from build123d import *

# Parameters (mm, degrees)
SKETCH1_R           = 1.25
BOSS_EXTRUDE1_DEPTH = 3


with BuildPart() as part:
    # Sketch1 → Boss-Extrude1 (new body)
    with BuildSketch(Plane.XY):
        with BuildLine():
            Line((-3.5, 0), (-3.5, -5))
            Line((-3.5, -5), (-2, -5))
            Line((-2, -5), (-2, -8))
            Line((-2, -8), (2, -8))
            Line((2, -8), (2, -5))
            Line((2, -5), (3.5, -5))
            Line((3.5, -5), (3.5, 0))
            ThreePointArc((3.5, 0), (0, 3.5), (-3.5, 0))
        make_face()
        Circle(SKETCH1_R, mode=Mode.SUBTRACT)
    extrude(amount=BOSS_EXTRUDE1_DEPTH)


solid = part.part
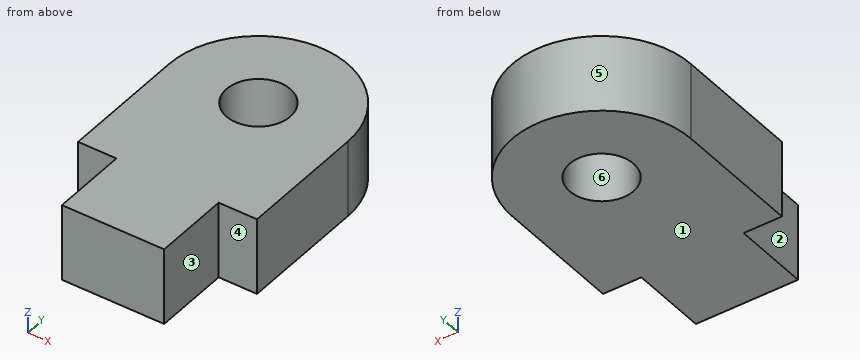
Source: CAD feature listing. Evaluate the final solid. Frame: model axes, mm. Face numbers are marked on the shaded views. A direction names the side the tool comes from. Round coordinates to 2 decimals unless told otherwise and drop trailing zeros. Order: outer loops, then holes, each group sorted by start corner. A loop starts at its lowest first (then second) coordinate and runs counter-clockwise, first axis right, second up. Notation, with made-up numbers: (82.5, 83.5) - (98.5, 83.5) arc R25 cw to (98.5, 116.5) - close; hole circle Ø7 at (-18.5, -17). An arc over 180 degrees is marked (long way). Use a Markdown table: item, result. Add a question column.
1. Mould query, pull axis X, two halves, no side actions, for the marked faces 4, 5 and 6. Classes: +X half, -X half, draft (parallel to the pull), parting line (faces both ways), or undercut.
2. Section query B-B (y = 0.25). Return the cut outline in (x, z), then the cut area to 3 significant figures.
3. Section query D-D (y = -7.25). Return the cut outline in (x, z), then the cut area to 3 significant figures.
4. Section query C-C (x = 0). Return the cut outline in (y, z), then the cut area to 3 significant figures.
5. Line query: probe 1 along Y at (x, z) = (0, 2); probe 2 along X at (y, z) = (-6, 2.05); probe 3 along Y at (x, z) = (1, 1.15). Output: solid intervals per line, ascending.
6. Section query A-A (z = 1.3). Return the cut outline in (x, y).
7. First-contact query: pin 1 (1.5 mm diameter, centred on x = -1, z = 1.5, fed in from +Y); pin 2 (1.6 mm diameter, centred on x = 2.5, z = 1, fed in from -Y); pin 3 (1.2 mm diameter, centred on x = -3, z = 1, fed in from -Y); pin 4 (1.5 mm diameter, centred on y = -6, z = 1, fed in from -X). Flat tips, straight axial feed; report the tip coordinate or a pass-through.
8. Set-up query: the marked faces 1, 2 and 3. Return all of +Z, -Z, +X, -X, +Y, -Y with unobstructed straight access to the full face (end or side cutting, diameter ignored); none if empty.
Derived:
| question | item | result |
|---|---|---|
| 1 | face 4 | draft |
| 1 | face 5 | parting line |
| 1 | face 6 | undercut |
| 2 | outline | (-3.49, 0) - (-1.22, 0) - (-1.22, 3) - (-3.49, 3) - close; (1.22, 0) - (3.49, 0) - (3.49, 3) - (1.22, 3) - close |
| 2 | area | 13.6 mm2 |
| 3 | outline | (-2, 0) - (2, 0) - (2, 3) - (-2, 3) - close |
| 3 | area | 12.0 mm2 |
| 4 | outline | (-8, 0) - (-1.25, 0) - (-1.25, 3) - (-8, 3) - close; (1.25, 0) - (3.5, 0) - (3.5, 3) - (1.25, 3) - close |
| 4 | area | 27.0 mm2 |
| 5 | probe 1 | -8 to -1.25, 1.25 to 3.5 |
| 5 | probe 2 | -2 to 2 |
| 5 | probe 3 | -8 to -0.75, 0.75 to 3.35 |
| 6 | outline | (-3.5, -5) - (-2, -5) - (-2, -8) - (2, -8) - (2, -5) - (3.5, -5) - (3.5, 0) arc R3.5 ccw to (-3.5, 0) - close; hole circle Ø2.5 at (0, 0) |
| 7 | pin 1 | y = 3.49 |
| 7 | pin 2 | y = -8 |
| 7 | pin 3 | y = -5 |
| 7 | pin 4 | x = -2 |
| 8 | face 1 | -Z, +X, -X, +Y, -Y |
| 8 | face 2 | +Z, -Z, -X, -Y |
| 8 | face 3 | +Z, -Z, +X, -Y |
